Could you check a few things on this drawing? It's one solid part, dimensions in mm from its lowest x, y, z. Coordinates: 2 decimals unless noted, no trailing zeros. Order: outer loops, then holes, each group sorted by start corner. A loop starts at its lowest first (then second) coordinate and runs counter-clockwise, first axis right, second up. Notation, with made-up numbers: M 58.25,-24 L 109.25,-24 A25 cw 109.25,11 Z; hole C 78.5,44 d4. An arc over 180 degrees is marked long. Write item = value, one per line. Start each with the question number.
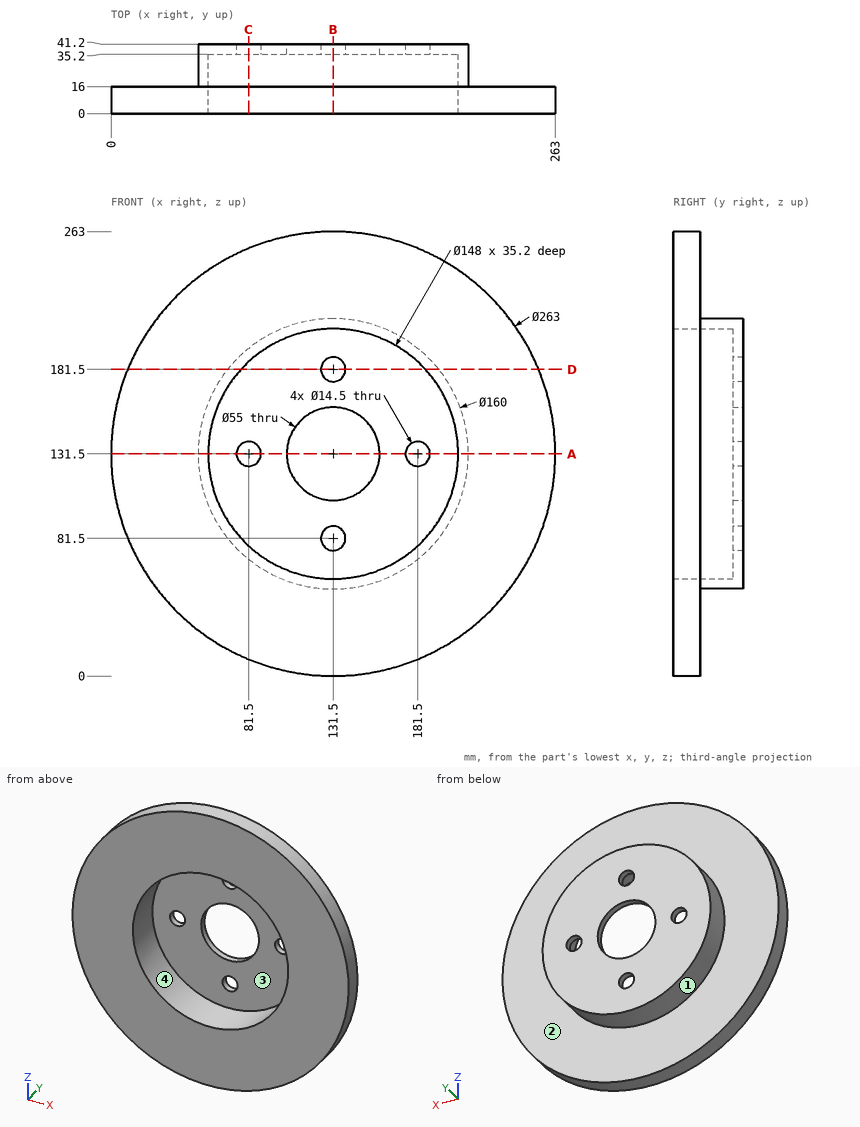
(1) Imagine slicing it at D-D on z = 181.5. List the corners of the cut face in (x, y) for me.
(2) Will these pins go through, and if not, where does the flat tip stop? P1, Ø4, axis at y = 15.5, z = 148.5, coming from the -X side; P2, Ø2, axis at x = 73.5, y = 17.5, coming from the +Z side; P3, Ø8, axis at x = 100, y = 10, coming from the -Z side.
(3) Imagine slicing it at C-C on x = 81.5. List the corners of the cut face in (y, z) for me, plus the area to 3 significant figures.
(4) Please list where these lines run through material, in increasing order: probe 1 along Z at (x, y) = (131.5, 37.55); probe 2 along Z at (x, y) = (131.5, 24); probe 3 along Z at (x, y) = (75.5, 9). Write a range as from..to.
(5) Imagine slicing it at B-B on x = 131.5. List the corners of the cut face in (y, z) for me, plus the area to 3 significant figures.
(6) Thinking about a two-plate mould opening in Z: for the marked faces 1, 2, 3 and 4, which applies, released by +Z, released by -Z, zero draft, split by the parting line, or undercut?
(7) Imagine slicing it at A-A on z = 131.5. List the corners of the cut face in (x, y) for me.
Response:
q1.outline = M 9.88,0 L 76.95,0 L 76.95,35.2 L 124.25,35.2 L 124.25,41.2 L 69.05,41.2 L 69.05,16 L 9.88,16 Z; M 138.75,35.2 L 186.05,35.2 L 186.05,0 L 253.12,0 L 253.12,16 L 193.95,16 L 193.95,41.2 L 138.75,41.2 Z
q2.P1 = 0.86
q2.P2 = 187.63
q2.P3 = 2.91
q3.outline = M 0,9.88 L 16,9.88 L 16,69.05 L 41.2,69.05 L 41.2,124.25 L 35.2,124.25 L 35.2,76.95 L 0,76.95 Z; M 0,186.05 L 35.2,186.05 L 35.2,138.75 L 41.2,138.75 L 41.2,193.95 L 16,193.95 L 16,253.12 L 0,253.12 Z
q3.area = 3,110 mm2
q4.probe_1 = 51.5..74.25, 88.75..104, 159..174.25, 188.75..211.5
q4.probe_2 = 51.5..57.5, 205.5..211.5
q4.probe_3 = 12.52..83.13, 179.87..250.48
q5.outline = M 0,0 L 16,0 L 16,51.5 L 41.2,51.5 L 41.2,74.25 L 35.2,74.25 L 35.2,57.5 L 0,57.5 Z; M 0,205.5 L 35.2,205.5 L 35.2,188.75 L 41.2,188.75 L 41.2,211.5 L 16,211.5 L 16,263 L 0,263 Z; M 35.2,88.75 L 41.2,88.75 L 41.2,104 L 35.2,104 Z; M 35.2,159 L 41.2,159 L 41.2,174.25 L 35.2,174.25 Z
q5.area = 2,530 mm2
q6.face_1 = split by the parting line
q6.face_2 = zero draft
q6.face_3 = undercut
q6.face_4 = undercut
q7.outline = M 0,0 L 57.5,0 L 57.5,35.2 L 74.25,35.2 L 74.25,41.2 L 51.5,41.2 L 51.5,16 L 0,16 Z; M 88.75,35.2 L 104,35.2 L 104,41.2 L 88.75,41.2 Z; M 159,35.2 L 174.25,35.2 L 174.25,41.2 L 159,41.2 Z; M 188.75,35.2 L 205.5,35.2 L 205.5,0 L 263,0 L 263,16 L 211.5,16 L 211.5,41.2 L 188.75,41.2 Z
